from build123d import *

# Parameters (mm, degrees)
SKETCH3_R = 4
P_L_DEPTH = 10


with BuildPart() as part:
    # Sketch1 → Revolve1 (revolve)
    with BuildSketch(Plane.XY):
        with BuildLine():
            Line((-30, 2), (19.8, 2))
            Line((19.8, 2), (20, 1.946410162))
            Line((20, 1.946410162), (20, 1.85))
            ThreePointArc((20, 1.85), (20.029289322, 1.779289322), (20.1, 1.75))
            Line((20.1, 1.75), (20.208578644, 1.75))
            ThreePointArc((20.208578644, 1.75), (20.246846987, 1.757612047), (20.279289322, 1.779289322))
            Line((20.279289322, 1.779289322), (20.5, 2))
            Line((20.5, 2), (31.5, 2))
            Line((31.5, 2), (32, 1.5))
            Line((32, 1.5), (32, 0))
            Line((32, 0), (-32, 0))
            Line((-32, 0), (-32, 4))
            Line((-32, 4), (-30, 4))
            Line((-30, 4), (-30, 2))
        make_face()
    revolve(axis=Axis((0, 0, 0), (1, 0, 0)))

    # Sketch3 → P-L (add)
    with BuildSketch(Plane.ZY.offset(32)):
        Circle(SKETCH3_R)
    extrude(amount=P_L_DEPTH)


solid = part.part
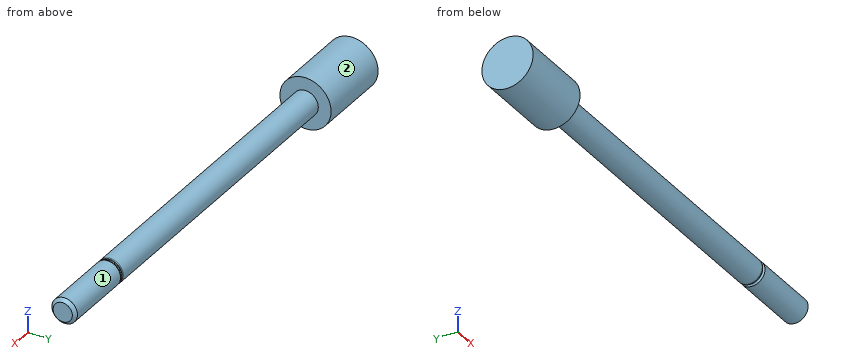
CAD build for the part. Positions are in the model's coordinates, mm. Face numbers are marked on the shaded views. A direction names the side the tool comes from. Round coordinates to 2 decimals unless told otherwise and drop trailing zeros. Order: outer loops, then holes, each group sorted by start corner. A loop starts at its lowest first (then second) coordinate and runs counter-clockwise, first axis right, second up. Notation, with made-up numbers: (42, 50.25) -> (67, 50.25) arc R29 cw to (67, 85.25) -> close; hole circle Ø8 at (4, 83.25). An arc over 180 degrees is marked (long way). Write item = value, one per line. Start each with the question number.
(1) Pin check, flat tips, straight feed: P1, Ø2, axis at x = 5, y = 2.5, coming from the +Z side; P2, Ø1.5, axis at x = -8.5, z = -2, coming from the +Y side; P3, Ø1, axis at y = -2, z = 2, coming from the +X side. Stop position of each tip, or through.
(2) Probe line 1 (X direction, y = -2.5, z = 3); line 2 (Y direction, x = -5.5, z = 0.75). List the from-to ranges inside material, lowest first. Write a range as [from, to].
(3) Cut at A-A, the plane z = 0. List the corners of the cut face in (x, y).
(4) Cut at D-D, the plane x = -37. List the corners of the cut face in (y, z), then the cut area to 3 significant figures.
(5) Which spindle directions (+Z, -Z, +X, -X, +Y, -Y) get a long thin tool onto all of the face, cutting with end or side? Do the marked faces 1 and 2. Say none if no direction does.
(6) Cut at C-C, the plane x = 15. List the corners of the cut face in (y, z).
Model answer:
q1.P1 = 1.32
q1.P2 = 1.56
q1.P3 = -30
q2.line_1 = [-42, -30]
q2.line_2 = [-1.85, 1.85]
q3.outline = (-42, -4) -> (-30, -4) -> (-30, -2) -> (19.8, -2) -> (20, -1.95) -> (20, -1.85) arc R0.1 cw to (20.1, -1.75) -> (20.21, -1.75) arc R0.1 cw to (20.28, -1.78) -> (20.5, -2) -> (31.5, -2) -> (32, -1.5) -> (32, 1.5) -> (31.5, 2) -> (20.5, 2) -> (20.28, 1.78) arc R0.1 cw to (20.21, 1.75) -> (20.1, 1.75) arc R0.1 cw to (20, 1.85) -> (20, 1.95) -> (19.8, 2) -> (-30, 2) -> (-30, 4) -> (-42, 4) -> close
q4.outline = circle Ø8 at (0, 0)
q4.area = 50.3 mm2
q5.face_1 = +X
q5.face_2 = +X, -X
q6.outline = circle Ø4 at (0, 0)
